from build123d import *

# Parameters (mm, degrees)
SKETCH1_R           = 60.325
BOSS_EXTRUDE1_DEPTH = 2.5
SKETCH2_R           = 4.064
CUT_EXTRUDE1_DEPTH  = 86.458827806
CUT_EXTRUDE4_DEPTH  = 86.458827806


with BuildPart() as part:
    # Sketch1 → Boss-Extrude1 (new, symmetric)
    with BuildSketch(Plane(origin=(0, 0, 0), x_dir=(0, 0, -1), z_dir=(1, 0, 0))):
        Circle(SKETCH1_R)
    extrude(amount=BOSS_EXTRUDE1_DEPTH, both=True)

    # Sketch2 → Cut-Extrude1 (cut, through all)
    with BuildSketch(Plane.ZY.offset(2.5)):
        with Locations((0, 50.342959834)):
            Circle(SKETCH2_R)
        with Locations((47.879, 15.556830136)):
            Circle(SKETCH2_R)
        with Locations((29.590849347, -40.728310053)):
            Circle(SKETCH2_R)
        with Locations((-29.590849347, -40.728310053)):
            Circle(SKETCH2_R)
        with Locations((-47.879, 15.556830136)):
            Circle(SKETCH2_R)
    extrude(amount=-CUT_EXTRUDE1_DEPTH, mode=Mode.SUBTRACT)

    # Sketch8 → Cut-Extrude4 (cut, through all)
    with BuildSketch(Plane(origin=(2.5, 0, 0), x_dir=(0, 0, -1), z_dir=(1, 0, 0))):
        with BuildLine():
            Line((0, 11.006403687), (-3, 11.006403687))
            Line((-3, 11.006403687), (-3, 8.006403687))
            ThreePointArc((-3, 8.006403687), (0, -8.55), (3, 8.006403687))
            Line((3, 8.006403687), (3, 11.006403687))
            Line((3, 11.006403687), (0, 11.006403687))
        make_face()
    extrude(amount=-CUT_EXTRUDE4_DEPTH, mode=Mode.SUBTRACT)


solid = part.part
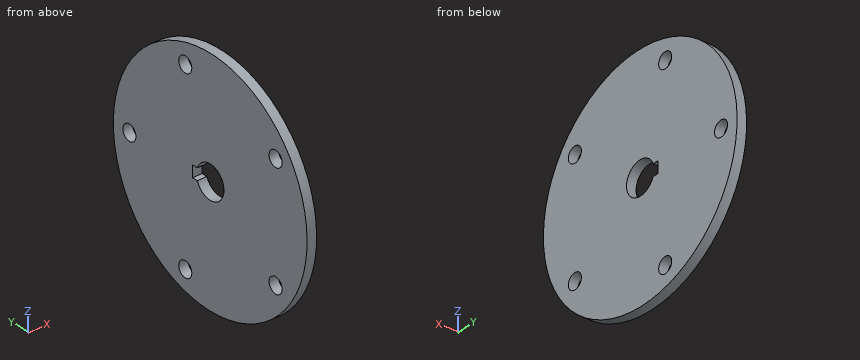
Here's how the part is built. I have some questions about the finished solid (model axes, mm). Coordinates: 2 decimals unless noted, no trailing zeros. Loops run counter-clockwise (first coordinate to the right, second up) from the corner with the lowest first, then second, coordinate; pieces in that order, holes last.
1. For P1, Ø1.5, axis at x = -1, y = 42, coming from the -Z side; P2, Ø1.5, axis at x = 0.5, y = -39, coming from the +Z side; P3, Ø0.9, axis at x = 0, y = 10, coming from the +Z side, each with a flat end and sliding along its axis, tell me the tip position at first contact or that it passes through.
2. Imagine slicing it at B-B, the plane y = 0. Please give me the cut outline in (x, z) (3 decimals).
3. I need wall thicknesses on L1, parallel to Z at x = -2.3, y = -41; L2, parallel to Z at x = -1.5, y = 50; L3, parallel to Y at x = 0.6, z = 27.5. Which ranges of each line are inside material? Lowest first, please.
4. Imagine slicing it at A-A, the plane z = 0. Please give me the cut outline in (x, y) (3 decimals), and give its area (3 significant figures).
5. Imagine slicing it at D-D, the plane y = -29. Please give me the cut outline in (x, z), and give its area (3 significant figures).
6. Imagine slicing it at C-C, the plane x = -0.9. Please give me the cut outline in (y, z) (3 decimals).
Taken from the geometry:
1. P1: stops at z = -44.02
1. P2: stops at z = 46.65
1. P3: stops at z = 59.56
2. outline: (-2.5, -60.325) - (2.5, -60.325) - (2.5, -8.55) - (-2.5, -8.55) - close; (-2.5, 8.55) - (2.5, 8.55) - (2.5, 60.325) - (-2.5, 60.325) - close
3. L1: z = -44.25 to -33.65, -25.54 to 25.54, 33.65 to 44.25
3. L2: z = -33.75 to -4.05, 4.05 to 33.75
3. L3: y = -53.69 to -44.21, -37.24 to 53.69
4. outline: (-2.5, -60.325) - (2.5, -60.325) - (2.5, -8.55) - (-2.5, -8.55) - close; (-2.5, 11.006) - (2.5, 11.006) - (2.5, 46.279) - (-2.5, 46.279) - close; (-2.5, 54.407) - (2.5, 54.407) - (2.5, 60.325) - (-2.5, 60.325) - close
4. area: 465 mm2
5. outline: (-2.5, -52.9) - (2.5, -52.9) - (2.5, 52.9) - (-2.5, 52.9) - close
5. area: 529 mm2
6. outline: circle Ø120.65 at (0, 0); hole circle Ø8.128 at (-40.728, -29.591); hole circle Ø8.128 at (-40.728, 29.591); hole (8.006, -3) - (11.006, -3) - (11.006, 3) - (8.006, 3) arc R8.55 ccw (long way) to start; hole circle Ø8.128 at (15.557, -47.879); hole circle Ø8.128 at (15.557, 47.879); hole circle Ø8.128 at (50.343, 0)
